from build123d import *

# Parameters (mm, degrees)
SKETCH1_R           = 20
BOSS_EXTRUDE1_DEPTH = 8
SKETCH2_R           = 7.5
CUT_EXTRUDE1_DEPTH  = 9
FILLET1_R           = 1


with BuildPart() as part:
    # Sketch1 → Boss-Extrude1 (new body)
    with BuildSketch(Plane(origin=(0, 0, 0), x_dir=(1, 0, 0), z_dir=(0, 1, 0))):
        Circle(SKETCH1_R)
    extrude(amount=BOSS_EXTRUDE1_DEPTH)

    # Sketch2 → Cut-Extrude1 (cut, through all)
    with BuildSketch(Plane(origin=(0, 8, 0), x_dir=(1, 0, 0), z_dir=(0, 1, 0))):
        Circle(SKETCH2_R)
    extrude(amount=-CUT_EXTRUDE1_DEPTH, mode=Mode.SUBTRACT)

    # Fillet1
    fillet1_edges = [part.edges().sort_by_distance(p)[0] for p in [
        (-7.5, 8, 0),
    ]]
    fillet(fillet1_edges, radius=FILLET1_R)


solid = part.part
The model under review builds one solid part; all positions refer to its coordinate system, in mm. Give positions to 0.01 mm unless a question says otherwise; leave off trailing zeros. Write each loop counter-clockwise with the first axis right and the second up, starting at its lowest first coordinate (ties: lowest second). Pieces come first, ordered by that corner, then holes. Notation, with made-up numbers: M 68,41 L 120,41 A18 ccw 120,60 Z; hole C 83,62.5 d4. An arc over 180 degrees is marked long. One line per question, with ' | ' between items. Start each with the question number.
Item 1: We need section C-C on y = 5.75. Write out the cut boundary in (x, z).
Item 2: We need section B-B on x = 0. Write out the cut boundary in (y, z).
Item 3: We need section A-A on z = 0. Write out the cut boundary in (x, y).
Item 4: Draft analysis for pull direction Z (two halves, no side actions). For faces 1 (the cylindrical face through (-7.493, 3.549, -0.33)), 2 (the flat face through (0, 0, 9)), 3 (the cylindrical face through (-4.336, 3.944, 19.524)), state which applies: released by +Z, released by -Z, zero draft, split by the parting line, or undercut.
Item 5: Wall thickness on line 1 (X direction, y = 3, z = 0); line 2 (Z direction, x = 4, y = 4.75): over which ranges is each line inside the solid? List them lowest first. Write a range as from..to.
Item 6: For pin 1 (1 mm diameter, centred on x = -10, y = 6, fed in from +Z); pin 2 (1.5 mm diameter, centred on y = 3, z = -4.5, fed in from -X); pin 3 (19.5 mm diameter, centred on x = 0, z = 0, fed in from -Y); pin 4 (1 mm diameter, centred on x = -0.5, y = 2, fed in from +Z), all flat-tipped, find the tip position at first contact; note any pin that passes through.
Item 7: We need section D-D on x = -17. Write out the cut boundary in (y, z).
Results found:
1) outline: C 0,0 d40; hole C 0,0 d15
2) outline: M 0,-20 L 8,-20 L 8,-8.5 A1 ccw 7,-7.5 L 0,-7.5 Z; M 0,7.5 L 7,7.5 A1 ccw 8,8.5 L 8,20 L 0,20 Z
3) outline: M -20,0 L -7.5,0 L -7.5,7 A1 ccw -8.5,8 L -20,8 Z; M 7.5,0 L 20,0 L 20,8 L 8.5,8 A1 ccw 7.5,7 Z
4) face 1: undercut | face 2: zero draft | face 3: split by the parting line
5) line 1: x = -20..-7.5, 7.5..20 | line 2: z = -19.6..-6.34, 6.34..19.6
6) pin 1: stops at z = 17.6 | pin 2: stops at x = -19.65 | pin 3: stops at y = 0 | pin 4: stops at z = 20
7) outline: M 0,-10.54 L 8,-10.54 L 8,10.54 L 0,10.54 Z
